Source: CAD feature listing. Evaluate the final solid. Frame: model axes, mm. Round coordinates to 2 decimals unless told otherwise and drop trailing zeros. Order: outer loops, then holes, each group sorted by start corner. A loop starts at its lowest first (then second) coordinate and runs counter-clockwise, first axis right, second up. Notation, with made-up numbers: (46.25, 53.25) -> (70.25, 53.25) arc R23 cw to (70.25, 81.25) -> close; hole circle Ø6 at (74.5, 49). An arc over 180 degrees is marked (long way). Answer as CSV lines item,"result".
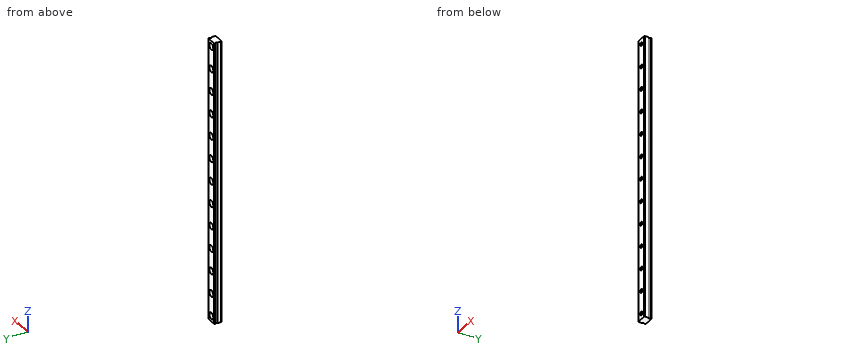
Autodesk Inventor part; units mm, degrees
ref_plane "YZ Plane" through (0, 0, 0) normal (1, 0, 0) x (0, 1, 0)
ref_plane "XZ Plane" through (0, 0, 0) normal (0, 1, 0) x (-1, 0, 0)
ref_plane "XY Plane" through (0, 0, 0) normal (0, 0, 1) x (1, 0, 0)
sketch "Sketch1" plane through (0, 0, 0) normal (0, 0, 1) x (1, 0, 0)
  line L0 (-4.5, -3.25) -> (4.5, -3.25)
  line L1 (4.5, -3.25) -> (4.5, 3.25)
  line L2 (4.5, 3.25) -> (-4.5, 3.25)
  line L3 (-4.5, 3.25) -> (-4.5, -3.25)
  line L4 (-4.5, -3.25) -> (4.5, 3.25) construction
  line L5 (4.5, -3.25) -> (-4.5, 3.25) construction
  circle A0 centre (-4.5, 1.25) radius 0.75
  circle A1 centre (4.5, 1.25) radius 0.75
  line L6 (-3.8126, 0.95) -> (3.8126, 0.95)
  line L7 (3.8126, 0.95) -> (3.8126, 1.55)
  line L8 (3.8126, 1.55) -> (-3.8126, 1.55)
  line L9 (-3.8126, 1.55) -> (-3.8126, 0.95)
  line L10 (-3.8126, 0.95) -> (3.8126, 1.55) construction
  line L11 (3.8126, 0.95) -> (-3.8126, 1.55) construction
  point P0 (0, 0)
  point P1 (0, 1.25)
  point P2 (-4.5, 2)
  point P3 (-4.5, 0.5)
  point P4 (4.5, 0.5)
  point P5 (4.5, 2)
  dimension "d2" = 1.5
  dimension "d0" = 9
  dimension "d1" = 6.5
  dimension "d3" = 4.5
  dimension "d4" = 0.6
extrude "Extrusion1" add sketch "Sketch1" along normal blind 250 contours L3 A0 L6 A1 L1 L0 | L3 L2 L1 A1 L8 A0 | A0 L8 A1 L6
chamfer "Chamfer1" distance 0.5 angle 45 4 edges at (-4.5, 3.25, 125) (-4.5, -3.25, 125) (4.5, 3.25, 125) (4.5, -3.25, 125)
sketch "Sketch2" plane through (-4, 3.25, 0) normal (0, 1, 0) x (1, 0, 0)
  line L0 (-0.5, 0) -> (-0.5, -250)
  line L1 (8, 0) -> (0, 0)
  point P0 (4, 0)
  point P1 (4, -5)
  point P2 (4, -25)
  point P3 (4, -45)
  point P4 (4, -65)
  point P5 (4, -85)
  point P6 (4, -105)
  point P7 (4, -125)
  point P8 (4, -145)
  point P9 (4, -165)
  point P10 (4, -185)
  point P11 (4, -205)
  point P12 (4, -225)
  point P13 (4, -245)
  dimension "d10" = 4.5
  dimension "d13" = 20
  dimension "d18" = 5
hole "Hole1" at (0, 3.25, 5) at (0, 3.25, 25) at (0, 3.25, 45) at (0, 3.25, 65) at (0, 3.25, 85) at (0, 3.25, 105) at (0, 3.25, 125) at (0, 3.25, 145) at (0, 3.25, 165) at (0, 3.25, 185) at (0, 3.25, 205) at (0, 3.25, 225) at (0, 3.25, 245) direction (0, -1, 0) diameter 3.3 depth 10 counterbore diameter 5.7 counterbore depth 4
properties part number "MGNRail250mm" material "Steel, Carbon"
1. Section query A-A on z = 91. Return loops of the section in (x, y).
Results below:
outline,"(-4.5, -2.75) -> (-4, -3.25) -> (4, -3.25) -> (4.5, -2.75) -> (4.5, 0.5) arc R0.75 cw to (4.5, 2) -> (4.5, 2.75) -> (4, 3.25) -> (-4, 3.25) -> (-4.5, 2.75) -> (-4.5, 2) arc R0.75 cw to (-4.5, 0.5) -> close"
2. Line query: L1, parallel to X at y = 2.2, z = 225; L2, parallel to X at y = -1.65, z = 245; L3, parallel to Y at x = 4.25, z = 142. Output: solid intervals per line, ascending. Write a range as [from, to].
Results below:
L1,"[-4.5, -2.85], [2.85, 4.5]"
L2,"[-4.5, -1.65], [1.65, 4.5]"
L3,"[-3, 0.54], [1.96, 3]"
3. Pin query (flat end, axial travel): pin 1 (2 mm diameter, centred on x = 0, z = 65, fed in from +Y); pin 2 (4.5 mm diameter, centred on x = 0, z = 225, fed in from +Y). Return the tip coordinate at first contact, or that it passes through.
Results below:
pin 1,"through"
pin 2,"y = -0.75"
